```python
from build123d import *

# Parameters (mm, degrees)
F0_W      = 69
F0_H      = 33.816832
F1_DEPTH  = 2
F2_W      = 30
F2_H      = 8.8
F3_DEPTH  = 25
F4_W      = 69
F4_H      = 20.016832
F5_DEPTH  = 25
F6_W      = 3
F6_H      = 5
F6_H_2    = 13.8
F7_DEPTH  = 5
F8_W      = 1
F8_H      = 4
F9_DEPTH  = 25
F10_W     = 1
F10_H     = 4
F11_DEPTH = 25


with BuildPart() as f1:
    # F0 (on Top) → F1 (new body)
    with BuildSketch(Plane.XY):
        with Locations((2.211537, -0.192308)):
            Rectangle(F0_W, F0_H)
    extrude(amount=F1_DEPTH)

    # F2 (on face) → F3 (cut)
    with BuildSketch(Plane(origin=(0, 0, 0), x_dir=(1, 0, 0), z_dir=(0, 0, -1))):
        with Locations((-17.288463, 12.700724)):
            Rectangle(F2_W, F2_H)
    extrude(amount=-F3_DEPTH, mode=Mode.SUBTRACT)

    # F4 (on face) → F5 (cut)
    with BuildSketch(Plane.XY.offset(2)):
        with Locations((2.211537, 6.707692)):
            Rectangle(F4_W, F4_H)
    extrude(amount=-F5_DEPTH, mode=Mode.SUBTRACT)

    # F6 (on face) → F7 (join)
    with BuildSketch(Plane(origin=(0, 0, 0), x_dir=(1, 0, 0), z_dir=(0, 0, -1))):
        with Locations((-30.788463, 5.800724)):
            Rectangle(F6_W, F6_H)
        with Locations((35.211537, 10.200724)):
            Rectangle(F6_W, F6_H_2)
    extrude(amount=F7_DEPTH)

    # F8 (on face) → F9 (cut)
    with BuildSketch(Plane.XZ.offset(17.100724)):
        with Locations((34.211537, -2)):
            Rectangle(F8_W, F8_H)
    extrude(amount=-F9_DEPTH, mode=Mode.SUBTRACT)

    # F10 (on face) → F11 (cut)
    with BuildSketch(Plane.XZ.offset(8.300724)):
        with Locations((-29.788463, -2)):
            Rectangle(F10_W, F10_H)
    extrude(amount=-F11_DEPTH, mode=Mode.SUBTRACT)


solid = f1.part
```
Verification items for the finished model (mm, model axes). A direction names the side the tool comes from. Coordinates: 2 decimals unless noted, no trailing zeros. Loops run counter-clockwise (first coordinate to the right, second up) from the corner with the lowest first, then second, coordinate; pieces in that order, holes last. Notation, with made-up numbers: (13, 44.5) -> (30, 44.5) arc R26 ccw to (30, 65.5) -> close; hole circle Ø4 at (-28.5, 35.5). An arc over 180 degrees is marked (long way). Answer in a Markdown table with one row per item.
1) Section check A-A (z = -2). Record the cut outline in (x, y).
The answers:
| item | result |
|---|---|
| outline | (-32.29, -8.3) -> (-30.29, -8.3) -> (-30.29, -3.3) -> (-32.29, -3.3) -> close; (34.71, -17.1) -> (36.71, -17.1) -> (36.71, -3.3) -> (34.71, -3.3) -> close |
2) Section check D-D (z = 1.25). Record the cut outline in (x, y), and give its area (3 significant figures).
The answers:
| item | result |
|---|---|
| outline | (-32.29, -8.3) -> (-2.29, -8.3) -> (-2.29, -17.1) -> (36.71, -17.1) -> (36.71, -3.3) -> (-32.29, -3.3) -> close |
| area | 688 mm2 |
3) Depth check by flat-ended pin: P1, Ø3.5, axis at x = -12.5, z = -2, coming from the -Y side; P2, Ø1, axis at y = -13.5, z = 0.5, coming from the -X side; P3, Ø1.2, axis at y = -11.5, z = -2.5, coming from the -X side. Enter the tip coordinate at first touch or a pass-through.
The answers:
| item | result |
|---|---|
| P1 | passes through |
| P2 | stops at x = -2.29 |
| P3 | stops at x = 34.71 |
4) Draft check along Z on faces 3 (the face through (35, -10, -5)), 4 (the face through (-32.288, -6, -1)), 5 (the face through (-30.288, -6, -2)), 6 (the face through (34.712, -10, -2)). Enter one of: released by +Z, released by -Z, zero draft, split by the parting line, or undercut.
The answers:
| item | result |
|---|---|
| face 3 | released by -Z |
| face 4 | zero draft |
| face 5 | undercut |
| face 6 | undercut |
5) Section check B-B (y = -5.5). Record the cut outline in (x, z).
The answers:
| item | result |
|---|---|
| outline | (-32.29, -5) -> (-29.29, -5) -> (-29.29, -4) -> (-30.29, -4) -> (-30.29, 0) -> (34.71, 0) -> (34.71, -4) -> (33.71, -4) -> (33.71, -5) -> (36.71, -5) -> (36.71, 2) -> (-32.29, 2) -> close |
6) Access from +Z, -Z, +X, -X, +Y, -Y to the whole of each face (thin tool, end or side, straight path). Record for faces 1 (the face through (9, -9, 2)), 2 (the face through (-21, -8.301, 1)).
The answers:
| item | result |
|---|---|
| face 1 | +Z, +X, -X, +Y, -Y |
| face 2 | +Z, -Z, -X, -Y |
7) Scan lines: line 1 along X through (y, z) = (-6.5, -2.75); line 2 along Z through (x, y) = (10.5, -8); line 3 along X through (y, z) = (-9.5, 1). Record each from-to range of solid material in increasing order. Write a range as from..to.
The answers:
| item | result |
|---|---|
| line 1 | x = -32.29..-30.29, 34.71..36.71 |
| line 2 | z = 0..2 |
| line 3 | x = -2.29..36.71 |
8) Section check C-C (x = 14.5). Record the cut outline in (y, z), and give its area (3 significant figures).
The answers:
| item | result |
|---|---|
| outline | (-17.1, 0) -> (-3.3, 0) -> (-3.3, 2) -> (-17.1, 2) -> close |
| area | 27.6 mm2 |
